CAD build for the part. Positions are in the model's coordinates, mm. Give positions to 0.01 mm unless a question says otherwise; leave off trailing zeros. Loops run counter-clockwise (first coordinate to the right, second up) from the corner with the lowest first, then second, coordinate; pieces in that order, holes last. Notation, with made-up numbers: M 34,29 L 67,29 A18 cw 67,53 Z; hole C 0.5,27 d10. An arc over 180 degrees is marked long. One line per question, with ' | ' between items.
```python
from build123d import *

# Parameters (mm, degrees)
F1_DEPTH = 0.889
F3_DEPTH = 0.381
F4_R     = 0.1778
F4_R_2   = 0.381
F5_DEPTH = 0.254


with BuildPart() as f1:
    # F0 (on Top) → F1 (new body)
    with BuildSketch(Plane.XY):
        Polygon((-24.947381, -12.216053), (-26.81388, -12.216053), (-26.81388, -15.690773), (23.98612, -15.690773), (23.98612, -12.216053), (-21.899363, -12.216053), (17.63612, 34.014853), (14.588101, 34.014853), align=None)
    extrude(amount=F1_DEPTH)

    # F2 (on face) → F3 (cut)
    with BuildSketch(Plane.XY.offset(0.889)):
        Polygon((-24.730167, -11.962053), (-24.947381, -12.216053), (-21.899363, -12.216053), (-21.682148, -11.962053), align=None)
    extrude(amount=-F3_DEPTH, mode=Mode.SUBTRACT)

    # F4 (on face) → F5 (join)
    with BuildSketch(Plane.XY.offset(0.889)):
        with Locations((-23.361975, -11.435006)):
            Circle(F4_R)
        with Locations((-22.067515, -11.142211)):
            Circle(F4_R)
        with Locations((-23.38488, -13.950873)):
            Circle(F4_R_2)
        with Locations((15.699644, 33.05497)):
            Circle(F4_R)
        with Locations((14.366657, 32.453973)):
            Circle(F4_R)
        with Locations((20.55712, -13.950873)):
            Circle(F4_R_2)
    extrude(amount=F5_DEPTH)


solid = f1.part
```
Item 1: Drop flat-ended pins along their axis: P1, Ø12.5, axis at x = 6, y = 19.5, coming from the +Z side; P2, Ø10, axis at x = -4.5, y = 13.5, coming from the -Z side. Give the stop position or say it passes through.
Conclusion:
P1: z = 0.89 | P2: z = 0
Item 2: Saw through at B-B on x = 1. Give the cut face in (y, z), and give its area (3 significant figures).
Conclusion:
outline: M -15.69,0 L -12.22,0 L -12.22,0.89 L -15.69,0.89 Z; M 14.56,0 L 18.13,0 L 18.13,0.89 L 14.56,0.89 Z | area: 6.26 mm²
Item 3: Saw through at C-C on y = -10. Give the cut face in (x, z), and give its area (3 significant figures).
Conclusion:
outline: M -23.05,0 L -20,0 L -20,0.89 L -23.05,0.89 Z | area: 2.71 mm²
Item 4: Drill centre lines: line 1 along Y through (x, z) = (10.5, 0.3); line 2 along Y through (x, z) = (-25, 0.1); line 3 along Y through (x, z) = (-1.5, 0.5). Where is each one in solid material? Low to high. Write a range as [from, to].
Conclusion:
line 1: [-15.69, -12.22], [25.67, 29.23] | line 2: [-15.69, -12.22] | line 3: [-15.69, -12.22], [11.64, 15.2]
Item 5: Saw through at A-A on z = 0.2. Give the cut face in (x, y), and give its area (3 significant figures).
Conclusion:
outline: M -26.81,-15.69 L 23.99,-15.69 L 23.99,-12.22 L -21.9,-12.22 L 17.64,34.01 L 14.59,34.01 L -24.95,-12.22 L -26.81,-12.22 Z | area: 317 mm²
